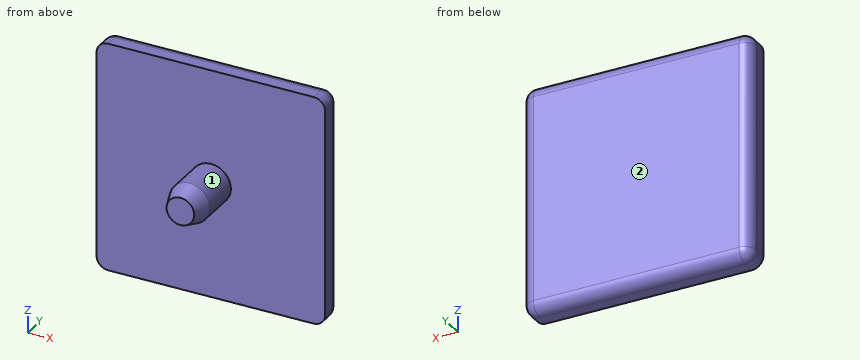
```python
from build123d import *

# Parameters (mm, degrees)
AUFSATZ_LINEAR_AUSTRAGEN1_DEPTH = 4.2
VERRUNDUNG1_R                   = 2
SKIZZE2_R                       = 3.5
AUFSATZ_LINEAR_AUSTRAGEN2_DEPTH = 10
FASE1_SIZE                      = 3
FASE1_SIZE2                     = 1.091910703


with BuildPart() as part:
    # Skizze1 → Aufsatz-Linear austragen1 (new body)
    with BuildSketch(Plane(origin=(0, 0, 0), x_dir=(1, 0, 0), z_dir=(0, 1, 0))):
        with BuildLine():
            Line((-20, -18), (-20, 18))
            ThreePointArc((-20, 18), (-19.414213562, 19.414213562), (-18, 20))
            Line((-18, 20), (18, 20))
            ThreePointArc((18, 20), (19.414213562, 19.414213562), (20, 18))
            Line((20, 18), (20, -18))
            ThreePointArc((20, -18), (19.414213562, -19.414213562), (18, -20))
            Line((18, -20), (-18, -20))
            ThreePointArc((-18, -20), (-19.414213562, -19.414213562), (-20, -18))
        make_face()
    extrude(amount=AUFSATZ_LINEAR_AUSTRAGEN1_DEPTH)

    # Verrundung1
    verrundung1_edges = [part.edges().sort_by_distance(p)[0] for p in [
        (-19.414213562, 4.2, 19.414213562),
        (0, 4.2, 20),
        (19.414213562, 4.2, 19.414213562),
        (20, 4.2, 0),
        (19.414213562, 4.2, -19.414213562),
        (0, 4.2, -20),
        (-19.414213562, 4.2, -19.414213562),
        (-20, 4.2, 0),
    ]]
    fillet(verrundung1_edges, radius=VERRUNDUNG1_R)

    # Skizze2 → Aufsatz-Linear austragen2 (add)
    with BuildSketch(Plane.XZ):
        with Locations(Location((0, 0, 0), (0, 0, 90))):
            Circle(SKIZZE2_R)
    extrude(amount=AUFSATZ_LINEAR_AUSTRAGEN2_DEPTH)

    # Fase1
    fase1_edges = [part.edges().sort_by_distance(p)[0] for p in [
        (0, -10, -3.5),
    ]]
    fase1_side = [part.faces().sort_by_distance(p)[0] for p in [
        (0, -5, -3.5),
    ]]
    chamfer(fase1_edges, length=FASE1_SIZE, length2=FASE1_SIZE2, reference=fase1_side[0])


solid = part.part
```
Could you check a few things on this model? Use its own coordinates, in mm. Face numbers are marked on the shaded views. A direction names the side the tool comes from. Give positions to 0.01 mm unless a question says otherwise; leave off trailing zeros. Loops run counter-clockwise (first coordinate to the right, second up) from the corner with the lowest first, then second, coordinate; pieces in that order, holes last. Notation, with made-up numbers: (76.5, -3) -> (118.5, -3) arc R4 ccw to (118.5, 4) -> close; hole circle Ø11 at (21.25, 9). An arc over 180 degrees is marked (long way). Put each result on its own line as item: value.
(1) Imagine slicing it at B-B on z = 0. Write out the boundary of the cut face in (x, y).
Computed:
outline: (-20, 0) -> (-3.5, 0) -> (-3.5, -7) -> (-2.41, -10) -> (2.41, -10) -> (3.5, -7) -> (3.5, 0) -> (20, 0) -> (20, 2.2) arc R2 ccw to (18, 4.2) -> (-18, 4.2) arc R2 ccw to (-20, 2.2) -> close
(2) I'm going to push flat-ended pins straight in: pin 1 Ø12 at (x, z) = (1, 3) entering from -Y; pin 2 Ø6 at (y, z) = (-5, 14) entering from -X; pin 3 Ø1.5 at (x, z) = (-13, 10.5) entering from -Y. Where does each tip first touch, or does it pass through?
Computed:
pin 1: y = -10
pin 2: through
pin 3: y = 0
(3) For the marked faces 1 and 2, which set-ups out of +Z, -Z, +X, -X, +Y, -Y let a thin tool reach every point of the face, with its end or its side?
Computed:
face 1: -Y
face 2: +Z, -Z, +X, -X, +Y
(4) Imagine slicing it at C-C on y = 3. Write out the boundary of the cut face in (x, z).
Computed:
outline: (-19.83, -18) arc R1.83 ccw to (-18, -19.83) -> (18, -19.83) arc R1.83 ccw to (19.83, -18) -> (19.83, 18) arc R1.83 ccw to (18, 19.83) -> (-18, 19.83) arc R1.83 ccw to (-19.83, 18) -> close
(5) Imagine slicing it at D-D on z = 17. Write out the boundary of the cut face in (x, y), plus the area to 3 significant figures.
Computed:
outline: (-20, 0) -> (20, 0) -> (20, 2.2) arc R2 ccw to (18, 4.2) -> (-18, 4.2) arc R2 ccw to (-20, 2.2) -> close
area: 166 mm^2
(6) Imagine slicing it at A-A on x = 0. Write out the boundary of the cut face in (y, z), plus the area to 3 significant figures.
Computed:
outline: (-10, -2.41) -> (-7, -3.5) -> (0, -3.5) -> (0, -20) -> (2.2, -20) arc R2 ccw to (4.2, -18) -> (4.2, 18) arc R2 ccw to (2.2, 20) -> (0, 20) -> (0, 3.5) -> (-7, 3.5) -> (-10, 2.41) -> close
area: 233 mm^2
(7) Please list where these lines run through material, in increasing order: probe 1 along Y at (x, z) = (13, -2); probe 2 along X at (y, z) = (-0.5, 0); probe 3 along Z at (x, y) = (-2, -1.5). Write a range as [from, to].
Computed:
probe 1: [0, 4.2]
probe 2: [-3.5, 3.5]
probe 3: [-2.87, 2.87]
